Can you work these out from the model? Positions are in its coordinate system, mm. Give positions to 0.01 mm unless a question says otherwise; leave off trailing zeros. Order: outer loops, then holes, each group sorted by start corner. A loop starts at its lowest first (then second) coordinate and runs counter-clockwise, first axis right, second up. Notation, with made-up numbers: (19.25, -8.75) - (61.25, -8.75) arc R13 cw to (61.25, 6.25) - close; hole circle Ø3 at (1.25, 14.5). An arc over 180 degrees is marked (long way). Return JSON: item names as keys, results as strings.
```python
from build123d import *

# Parameters (mm, degrees)
F1_DEPTH = 25.4
F3_DEPTH = 25.4


with BuildPart() as f1:
    # F0 (on Front) → F1 (new body)
    with BuildSketch(Plane.XZ):
        with BuildLine():
            Line((0, 20.139488), (0, 0))
            Line((0, 0), (57.15, 0))
            Line((57.15, 0), (57.15, 32.839488))
            Line((57.15, 32.839488), (12.7, 32.839488))
            ThreePointArc((12.7, 32.839488), (3.719744, 29.119744), (0, 20.139488))
        make_face()
    extrude(amount=F1_DEPTH)

    # F2 (on face) → F3 (cut)
    with BuildSketch(Plane.XZ.offset(25.4)):
        with BuildLine():
            Line((57.15, 32.839488), (34.925, 32.839488))
            ThreePointArc((34.925, 32.839488), (42.511039, 19.856363), (57.15, 16.419744))
            Line((57.15, 16.419744), (57.15, 32.839488))
        make_face()
    extrude(amount=-F3_DEPTH, mode=Mode.SUBTRACT)


solid = f1.part
```
1. Thinking about a two-plate mould opening in X: for faces 1 (the face through (42.338, -12.878, 19.986)), 2 (the face through (57.15, -13, 8)), 3 (the face through (0, -13, 10)), 4 (the face through (24, -13, 32.839)), which applies, +X half, -X half, draft (parallel to the pull), parting line (faces both ways), or undercut?
Checks:
{"face 1": "undercut", "face 2": "+X half", "face 3": "-X half", "face 4": "draft"}
2. Suppose I cut it at C-C (x = 53.5). List the corners of the cut face in (y, z) for me, plus the area to 3 significant figures.
Checks:
{"outline": "(-25.4, 0) - (0, 0) - (0, 16.13) - (-25.4, 16.13) - close", "area": "410 mm^2"}
3. Suppose I cut it at B-B (z = 23). List the corners of the cut face in (x, y) for me, plus the area to 3 significant figures.
Checks:
{"outline": "(0.33, -25.4) - (39.18, -25.4) - (39.18, 0) - (0.33, 0) - close", "area": "987 mm^2"}
4. For pin 1 Ø1 at (y, z) = (-14, 23) entering from +X, with a flat end and sliding along its axis, tell me the tip position at first contact or that it passes through.
Checks:
{"pin 1": "x = 39.61"}
5. Suppose I cut it at A-A (y = -4.25). List the corners of the cut face in (x, z) for me (3 decimals), plus the area to 3 significant figures.
Checks:
{"outline": "(0, 0) - (57.15, 0) - (57.15, 16.42) arc R19.05 cw to (34.925, 32.839) - (12.7, 32.839) arc R12.7 ccw to (0, 20.139) - close", "area": "1,550 mm^2"}
6. If I drill on L1, parallel to Z at x = 3, y = -24; L2, parallel to Z at x = 47, y = -24.5; L3, parallel to X at y = -20.25, z = 22.5, over which ranges is the centre line in solid material (lowest first)? Write a range as [from, to].
Checks:
{"L1": "[0, 28.34]", "L2": "[0, 17.4]", "L3": "[0.22, 39.61]"}
